```python
from build123d import *

# Parameters (mm, degrees)
F1_DEPTH = 6.35


with BuildPart() as f1:
    # F0 (on Top) → F1 (new body)
    with BuildSketch(Plane.XY):
        with BuildLine():
            ThreePointArc((-87.154024, 15.798011), (-90.694749, 13.563629), (-92.075, 9.610896))
            Line((-92.075, 9.610896), (-92.075, -8.65))
            ThreePointArc((-92.075, -8.65), (-90.215128, -13.140128), (-85.725, -15))
            Line((-85.725, -15), (-50.8, -15))
            ThreePointArc((-50.8, -15), (-14.878976, -29.878976), (0, -65.8))
            Line((0, -65.8), (0, -69.2))
            ThreePointArc((0, -69.2), (14.878976, -105.121024), (50.8, -120))
            Line((50.8, -120), (64.575, -120))
            ThreePointArc((64.575, -120), (69.065128, -118.140128), (70.925, -113.65))
            Line((70.925, -113.65), (70.925, -87.784507))
            ThreePointArc((70.925, -87.784507), (70.405264, -85.268454), (68.931135, -83.16427))
            ThreePointArc((68.931135, -83.16427), (33.041556, 0), (68.931135, 83.16427))
            ThreePointArc((68.931135, 83.16427), (70.405264, 85.268454), (70.925, 87.784507))
            Line((70.925, 87.784507), (70.925, 113.65))
            ThreePointArc((70.925, 113.65), (69.065128, 118.140128), (64.575, 120))
            Line((64.575, 120), (22.225, 120))
            ThreePointArc((22.225, 120), (17.734872, 118.140128), (15.875, 113.65))
            Line((15.875, 113.65), (15.875, 81.9))
            ThreePointArc((15.875, 81.9), (14.015128, 77.409872), (9.525, 75.55))
            Line((9.525, 75.55), (-9.525, 75.55))
            ThreePointArc((-9.525, 75.55), (-14.015128, 77.409872), (-15.875, 81.9))
            Line((-15.875, 81.9), (-15.875, 113.65))
            ThreePointArc((-15.875, 113.65), (-17.734872, 118.140128), (-22.225, 120))
            Line((-22.225, 120), (-85.725, 120))
            ThreePointArc((-85.725, 120), (-90.215128, 118.140128), (-92.075, 113.65))
            Line((-92.075, 113.65), (-92.075, 95.389104))
            ThreePointArc((-92.075, 95.389104), (-90.694749, 91.436371), (-87.154024, 89.201989))
            ThreePointArc((-87.154024, 89.201989), (-57.962776, 52.5), (-87.154024, 15.798011))
        make_face()
    extrude(amount=-F1_DEPTH)


solid = f1.part
```
Can you work these out from the model? Positions are in its coordinate system, mm. A direction names the side the tool comes from. Coordinates: 2 decimals unless noted, no trailing zeros. Loops run counter-clockwise (first coordinate to the right, second up) from the corner with the lowest first, then second, coordinate; pieces in that order, holes last.
1) Which directions (+Z, -Z, +X, -X, +Y, -Y) give clear straight access to the entire face, cutting with the end or side of a thin tool? Please do faces 4 (the cylindrical face through (17.785, 118.189, -3.131)), 5 (the cylindrical face through (-90.73, 91.48, -3.13)), 6 (the cylindrical face through (14.486, -104.724, -3.131)).
2) I need wall thicknesses on probe 1 along Y at (x, z) = (50, -3.25); probe 2 along Y at (x, z) = (54.5, -3.25); probe 3 along X at (y, z) = (-99, -2.75) (3 decimals). Which ranges of each line are inside material? Lowest first, please.
3) Thinking about a two-plate mould opening in Y: for faces 1 (the flat face through (-15.875, 98, -3)), 2 (the cylindrical face through (-13.965, 77.361, -3.131)), 3 (the cylindrical face through (70.42, -85.3, -3.13)), which applies, pulls with the +Y half, pulls with the -Y half, needs draft (parallel to the pull), parting line crosses it, or undercut?
4) Imagine slicing it at D-D on x = 3.5. List the corners of the cut face in (y, z) for me.
5) For pin 1 (1 mm diameter, centred on y = -67.5, z = -3, fed in from -X); pin 2 (3 mm diameter, centred on x = -76, z = -3, fed in from -Y); pin 3 (3 mm diameter, centred on x = 0, z = -4.5, fed in from +Y), each with a flat end and sliding along its axis, tell me the tip position at first contact or that it passes through.
6) Imagine slicing it at C-C on y = -4.5. List the corners of the cut face in (x, z) for me (3 decimals), plus the area to 3 significant figures.
7) Imagine slicing it at A-A on x = 56. List the corners of the cut face in (y, z) for me, plus the area to 3 significant figures.
Completed:
1. face 4: +Z, -Z, +Y
1. face 5: +Z, -Z, -X
1. face 6: +Z, -Z, -X, -Y
2. probe 1: y = -119.99 to -59.91, 59.91 to 120
2. probe 2: y = -120 to -66.67, 66.67 to 120
2. probe 3: x = 9.659 to 70.925
3. face 1: needs draft
3. face 2: pulls with the +Y half
3. face 3: undercut
4. outline: (-87.73, -6.35) - (75.55, -6.35) - (75.55, 0) - (-87.73, 0) - close
5. pin 1: stops at x = 0
5. pin 2: stops at y = -15
5. pin 3: stops at y = 75.55
6. outline: (-92.075, -6.35) - (33.13, -6.35) - (33.13, 0) - (-92.075, 0) - close
6. area: 795 mm2
7. outline: (-120, -6.35) - (-68.71, -6.35) - (-68.71, 0) - (-120, 0) - close; (68.71, -6.35) - (120, -6.35) - (120, 0) - (68.71, 0) - close
7. area: 651 mm2
